from build123d import *

# Parameters (mm, degrees)
BOSS_EXTRUDE1_DEPTH = 9.5
BOSS_EXTRUDE2_DEPTH = 19
BOSS_EXTRUDE3_DEPTH = 9.5
SKETCH4_R           = 9.5
CUT_EXTRUDE1_DEPTH  = 138.588150993
BOSS_EXTRUDE4_START = 6
SKETCH4_2_R         = 9.5
BOSS_EXTRUDE4_DEPTH = 50


with BuildPart() as part:
    # Sketch1 → Boss-Extrude1 (new body)
    with BuildSketch(Plane(origin=(0, 0, 0), x_dir=(1, 0, 0), z_dir=(0, 1, 0))):
        with BuildLine():
            ThreePointArc((107.722957073, -0.512015135), (-0.194984925, 25.004261154), (-108.658621874, 1.917424631))
            ThreePointArc((-108.658621874, 1.917424631), (-120.938659261, -31.236770908), (-87.784463723, -43.516808294))
            ThreePointArc((-87.784463723, -43.516808294), (-0.756328147, -24.992587685), (85.83395733, -45.466121624))
            ThreePointArc((85.83395733, -45.466121624), (119.255510446, -33.933568251), (107.722957073, -0.512015135))
        make_face()
    extrude(amount=BOSS_EXTRUDE1_DEPTH)

    # Sketch2 → Boss-Extrude2 (add)
    with BuildSketch(Plane(origin=(0, 9.5, 0), x_dir=(1, 0, 0), z_dir=(0, 1, 0))):
        with BuildLine():
            ThreePointArc((-32.906939519, -27.189629795), (-16.497958857, -25.426692254), (0, -25.00248869))
            Line((0, -25.00248869), (0, 25.001996795))
            ThreePointArc((0, 25.001996795), (-23.040926793, 24.228013528), (-45.915742347, 21.359883308))
            Line((-45.915742347, 21.359883308), (-32.906939519, -27.189629795))
        make_face()
        with BuildLine():
            Line((0, 25.001996795), (0, -25.00248869))
            ThreePointArc((0, -25.00248869), (16.389471048, -25.911302862), (32.651934744, -28.141320571))
            Line((32.651934744, -28.141320571), (45.630544935, 20.295512075))
            ThreePointArc((45.630544935, 20.295512075), (22.922161915, 23.685074324), (0, 25.001996795))
        make_face()
    extrude(amount=BOSS_EXTRUDE2_DEPTH)

    # Sketch3 → Boss-Extrude3 (add)
    with BuildSketch(Plane(origin=(0, 28.5, 0), x_dir=(1, 0, 0), z_dir=(0, 1, 0))):
        with BuildLine():
            ThreePointArc((107.722957073, -0.512015135), (-0.194984925, 25.004261154), (-108.658621874, 1.917424631))
            ThreePointArc((-108.658621874, 1.917424631), (-120.938659261, -31.236770908), (-87.784463723, -43.516808294))
            ThreePointArc((-87.784463723, -43.516808294), (-0.756328147, -24.992587685), (85.83395733, -45.466121624))
            ThreePointArc((85.83395733, -45.466121624), (119.255510446, -33.933568251), (107.722957073, -0.512015135))
        make_face()
    extrude(amount=BOSS_EXTRUDE3_DEPTH)

    # Sketch4 → Cut-Extrude1 (cut, through all)
    with BuildSketch(Plane(origin=(0, 38, 0), x_dir=(1, 0, 0), z_dir=(0, 1, 0))):
        with Locations(Location((-98.221542799, -20.799691832, 0), (0, 0, 270))):
            Circle(SKETCH4_R)
        with Locations(Location((96.778457201, -22.989068379, 0), (0, 0, 270))):
            Circle(SKETCH4_R)
    extrude(amount=-CUT_EXTRUDE1_DEPTH, mode=Mode.SUBTRACT)

    # Sketch4_2 → Boss-Extrude4 (add)
    with BuildSketch(Plane(origin=(0, 38, 0), x_dir=(1, 0, 0), z_dir=(0, 1, 0)).offset(BOSS_EXTRUDE4_START)):
        with Locations(Location((-98.221542799, -20.799691832, 0), (0, 0, 270))):
            Circle(SKETCH4_2_R)
        with Locations(Location((96.778457201, -22.989068379, 0), (0, 0, 270))):
            Circle(SKETCH4_2_R)
    extrude(amount=-BOSS_EXTRUDE4_DEPTH)


solid = part.part
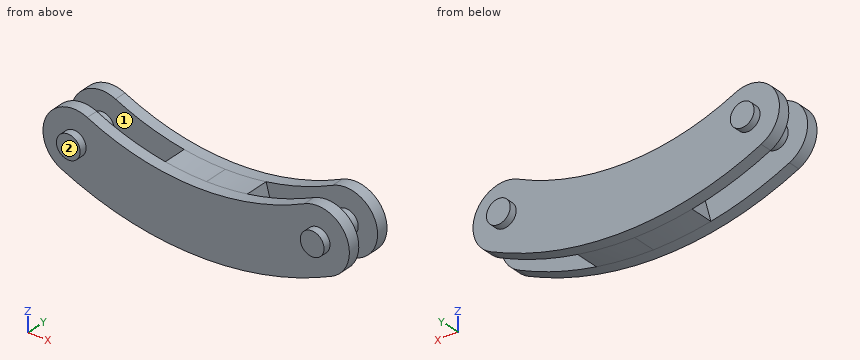
Design review of the part built by this model. Coordinates are the model's own, in mm. Face numbers are marked on the shaded views. Give positions to 0.01 mm unless a question says otherwise; leave off trailing zeros. Loops run counter-clockwise (first coordinate to the right, second up) from the corner with the lowest first, then second, coordinate; pieces in that order, holes last. Notation, with made-up numbers: (60.5, -31) - (81.5, -31) arc R10 ccw to (81.5, -22) - close; hole circle Ø2 at (-16, 12). An arc over 180 degrees is marked (long way). Write item = value, one per line.
1) Take a section at D-D on x = 3. State the section outline as (y, z) points.
Result sheet:
outline = (0, -24.95) - (38, -24.95) - (38, 25.07) - (0, 25.07) - close
2) To check wall thickness, follow line 1 (Y direction, x = 102.5, z = 11.5); line 2 (X direction, y = 18, z = 19); line 3 (X direction, y = -1.5, z = 25.5). State the ranges of each line that lie inside material, in increasing order.
Result sheet:
line_1 = 0 to 9.5, 28.5 to 38
line_2 = -107.55 to -88.89, -35.1 to 35.1, 88.16 to 105.4
line_3 = -106.48 to -89.97, 87.62 to 105.94
3) Take a section at A-A on x = 49. State the section outline as (y, z) points.
Result sheet:
outline = (0, -19.61) - (9.5, -19.61) - (9.5, 31.76) - (0, 31.76) - close; (28.5, -19.61) - (38, -19.61) - (38, 31.76) - (28.5, 31.76) - close
4) Take a section at B-B on y = 18. State the section outline as (x, z) points, and give its area (3 significant figures).
Result sheet:
outline = circle Ø19 at (-98.22, 20.8); (-45.92, -21.36) arc R253 ccw to (45.63, -20.3) - (32.65, 28.14) arc R203 cw to (-32.91, 27.19) - close; circle Ø19 at (96.78, 22.99)
area = 4,510 mm2
5) Draft analysis for pull direction X (two halves, no side actions). For the marked faces 1 and 2, state which applies: +X half, -X half, draft (parallel to the pull), parting line (faces both ways), or undercut.
Result sheet:
face_1 = undercut
face_2 = draft
6) Take a section at C-C on z = 39. State the section outline as (x, y) points.
Result sheet:
outline = (-115.36, 0) - (-77.17, 0) - (-77.17, 9.5) - (-115.36, 9.5) - close; (-115.36, 28.5) - (-77.17, 28.5) - (-77.17, 38) - (-115.36, 38) - close; (71.1, 0) - (115.98, 0) - (115.98, 9.5) - (71.1, 9.5) - close; (71.1, 28.5) - (115.98, 28.5) - (115.98, 38) - (71.1, 38) - close
7) Clearance check with flat-ended pins moving along their axes: pin 1 Ø22 at (x, z) = (-55, 4.5) entering from +Y; pin 2 Ø2 at (x, y) = (-5, 8) entering from +Z; pin 3 Ø5 at (y, z) = (31, 37) entering from +X. State where each tip first meets the part, or that it passes through.
Result sheet:
pin_1 = 38
pin_2 = 25
pin_3 = 118.97
